from build123d import *

# Parameters (mm, degrees)
F0_W          = 2405
F0_H          = 50
F1_DEPTH      = 15
F1_DEPTH_BACK = 15
F2_W          = 60
F2_H          = 30
F3_DEPTH      = 5
F4_W          = 60
F4_H          = 30
F5_DEPTH      = 5
F6_R          = 6
F7_DEPTH      = 5
F9_DEPTH      = 5
F10_DEPTH     = 5
F11_DEPTH     = 5


# Not quite as in the source:
# - a feature of the source that left no trace in its solid (it failed there, or was rolled back) is left out
# - a pattern or mirror of a feature is missing from the dataset's text; its kind, count and spacing are read off the source's solid
# - a feature names something its author has since deleted; it is built from what else it names


with BuildPart() as f1:
    # F0 (on Front) → F1 (new body, two sides)
    with BuildSketch(Plane.XZ) as f1_sk:
        Rectangle(F0_W, F0_H)
    extrude(amount=F1_DEPTH)
    extrude(f1_sk.sketch, amount=-F1_DEPTH_BACK)

    # F2 (on face) → F3 (join)
    with BuildSketch(Plane(origin=(0, 0, -25), x_dir=(1, 0, 0), z_dir=(0, 0, -1))):
        with Locations((-1172.5, -30)):
            Rectangle(F2_W, F2_H)
        Polygon((-1142.5, 15), (-1202.5, 15), (-1202.5, 0), (-1202.5, -15), (-1142.5, -15), align=None)
    extrude(amount=F3_DEPTH)

    # F4 (on face) → F5 (join)
    with BuildSketch(Plane(origin=(0, 0, -25), x_dir=(1, 0, 0), z_dir=(0, 0, -1))):
        with Locations((1172.5, -30)):
            Rectangle(F4_W, F4_H)
        Polygon((1202.5, 0), (1202.5, 15), (1142.5, 15), (1142.5, -15), (1202.5, -15), align=None)
    extrude(amount=F5_DEPTH)

    # F6 (on face) → F7 (cut, through all)
    with BuildSketch(Plane(origin=(0, 0, -30), x_dir=(1, 0, 0), z_dir=(0, 0, -1))):
        with Locations((1167.5, -30)):
            Circle(F6_R)
    extrude(amount=-F7_DEPTH, mode=Mode.SUBTRACT)

    # F8 (on face) → F9 (cut, through all)
    with BuildSketch(Plane(origin=(0, 0, -30), x_dir=(1, 0, 0), z_dir=(0, 0, -1))):
        with BuildLine():
            ThreePointArc((-1173.5, -30), (-1167.5, -36), (-1161.5, -30))
            ThreePointArc((-1161.5, -30), (-1167.5, -24), (-1173.5, -30))
        make_face()
    extrude(amount=-F9_DEPTH, mode=Mode.SUBTRACT)

    # F10 (add): faces of the model
    f10_faces = [f1.faces().sort_by_distance(p)[0] for p in [
        (1172.5, 44.3291796068, -25),
        (-1201.8291796068, 30, -25),
    ]]
    extrude(f10_faces, amount=F10_DEPTH)

    # F11 (cut): faces of the model
    f11_faces = [f1.faces().sort_by_distance(p)[0] for p in [
        (-1172.6621744947, 14.5134765159, -30),
        (1172.6621744947, 14.5134765159, -30),
    ]]
    extrude(f11_faces, amount=-F11_DEPTH, mode=Mode.SUBTRACT)

    # F14: sweep along a path in F13
    with BuildLine(Plane.XY) as f14_path:
        Line((1122.5, 15), (1122.5, 105))
        ThreePointArc((1122.5, 105), (1119.5710678119, 112.0710678119), (1112.5, 115))
        Line((1112.5, 115), (-1112.5, 115))
        ThreePointArc((-1112.5, 115), (-1119.5710678119, 112.0710678119), (-1122.5, 105))
        Line((-1122.5, 105), (-1122.5, 15))
    # F12 (on face) → F14 (sweep)
    with BuildSketch(Plane(origin=(0, 15, 0), x_dir=(-1, 0, 0), z_dir=(0, 1, 0))):
        with BuildLine():
            Line((-1122.5, 0), (-1122.5, 6))
            ThreePointArc((-1122.5, 6), (-1126.7426406871, -4.2426406871), (-1116.5, 0))
            Line((-1116.5, 0), (-1122.5, 0))
        make_face()
        with BuildLine():
            ThreePointArc((-1116.5, 0), (-1118.2573593129, 4.2426406871), (-1122.5, 6))
            Line((-1122.5, 6), (-1122.5, 0))
            Line((-1122.5, 0), (-1116.5, 0))
        make_face()
    sweep(path=f14_path.line)

    # F15: sweep along a path in F13
    with BuildLine(Plane.XY) as f15_path:
        Line((-561.25, 115), (-561.25, 15))
    # F12 (on face) → F15 (sweep)
    with BuildSketch(Plane(origin=(0, 15, 0), x_dir=(-1, 0, 0), z_dir=(0, 1, 0))):
        with BuildLine():
            ThreePointArc((567.25, 0), (561.25, 6), (555.25, 0))
            Line((555.25, 0), (567.25, 0))
        make_face()
        with BuildLine():
            Line((567.25, 0), (555.25, 0))
            ThreePointArc((555.25, 0), (561.25, -6), (567.25, 0))
        make_face()
    f15 = sweep(path=f15_path.line)

    # F15_copies: F15 across plane
    add(f15.mirror(Plane(origin=(-280.625, 0, 0), x_dir=(0, 0, 1), z_dir=(1, 0, 0))))

    # F17: sweep along a path in F13
    with BuildLine(Plane.XY) as f17_path:
        Line((561.25, 115), (561.25, 15))
    # F12 (on face) → F17 (sweep)
    with BuildSketch(Plane(origin=(0, 15, 0), x_dir=(-1, 0, 0), z_dir=(0, 1, 0))):
        with BuildLine():
            ThreePointArc((-555.25, 0), (-561.25, 6), (-567.25, 0))
            Line((-567.25, 0), (-555.25, 0))
        make_face()
        with BuildLine():
            Line((-555.25, 0), (-567.25, 0))
            ThreePointArc((-567.25, 0), (-561.25, -6), (-555.25, 0))
        make_face()
    sweep(path=f17_path.line)


solid = f1.part
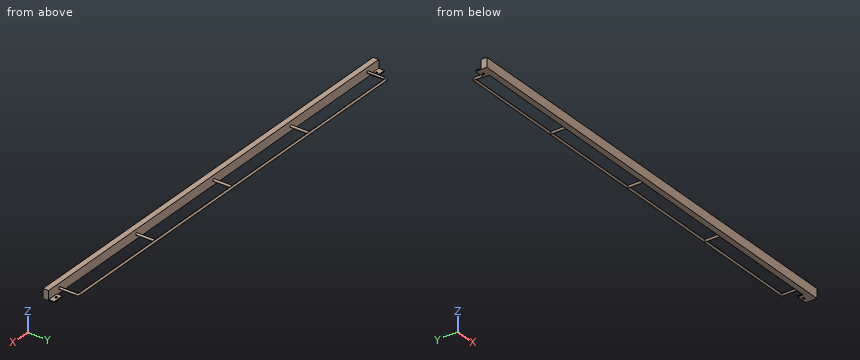
Geometry: final body of the model. Coordinates: model frame, mm. Give positions to 0.01 mm unless a question says otherwise; leave off trailing zeros. Loops run counter-clockwise (first coordinate to the right, second up) from the corner with the lowest first, then second, coordinate; pieces in that order, holes last. Notation, with made-up numbers: (-16, -40) - (21, -40) arc R12 cw to (21, -24) - close; hole circle Ø10 at (88, 30.25). An arc over 180 degrees is marked (long way). One line per question, with ' | ' between items. Start each with the question number.
(1) Ray query, line 1 (X direction, y = 30, z = -21); line 2 (Y direction, x = -1167.5, z = -22.9); line 3 (Y direction, x = -104.5, z = 1). Return the intervals inside material, ascending. Write a range as from..to.
(2) Contact query for flat-ended pins moving along their axis: pin 1 (1.5 mm diameter, centred on x = -1159, z = -23, fed in from +Y); pin 2 (5 mm diameter, centred on y = 23.5, z = -6, fed in from +X); pin 3 (15 mm diameter, centred on x = -31, z = -4, fed in from +Y); pin 4 (9 mm diameter, centred on x = 1174.5, y = 31, fed in from +Z). Output: stop coordinate, or through.
(3) Section query A-A on x = 388. Return loops of the section in (y, z), then the cut area to 3 significant figures.
(4) Section query B-B on y = 85.5. Return loops of the section in (x, z).
The answers:
1) line 1: -1202.5..-1173.5, -1161.5..-1142.5, 1142.5..1161.5, 1173.5..1202.5 | line 2: -15..24, 36..45 | line 3: -15..15, 109.08..120.92
2) pin 1: y = 45 | pin 2: x = 1127.37 | pin 3: y = 121 | pin 4: z = -20
3) outline: (-15, -25) - (15, -25) - (15, 25) - (-15, 25) - close; circle Ø12 at (115, 0) | area: 1,610 mm2
4) outline: circle Ø12 at (-1122.5, 0); circle Ø12 at (-561.25, 0); circle Ø12 at (0, 0); circle Ø12 at (561.25, 0); circle Ø12 at (1122.5, 0)
